CAD build for the part. Positions are in the model's coordinates, mm. Round coordinates to 2 decimals unless told otherwise and drop trailing zeros. Order: outer loops, then holes, each group sorted by start corner. A loop starts at its lowest first (then second) coordinate and runs counter-clockwise, first axis right, second up. Notation, with made-up numbers: (35.25, 7) -> (42.25, 7) arc R33 cw to (42.25, 44) -> close; hole circle Ø4 at (-31.75, -12). An arc over 180 degrees is marked (long way). Return JSON: item names as keys, results as strings. Group by question number.
Q1. Mould opens along Y. For faces 1 (the cylindrical face through (-4.119, 213.452, 1.479)), 2 (the flat face through (-9, 4, 0)) say: +Y half, -Y half, draft (parallel to the pull), parting line (faces both ways), or undercut.
Q2. Cut at B-B (x = 0). Write the cut outline in (y, z).
Q3. Cut at A-A (y = 232). Write the cut outline in (x, z), then the cut area to 3 significant figures.
Q4. Probe line 1 along Y through (x, z) = (-101, 2.2); line 2 along X through (y, z) = (-180, 0.8); line 3 along Y through (x, z) = (615, 2.15). List the from-to ranges inside material, lowest first.
Q5. Flat gauge pins, fed straight in: pin 1 (8 mm diameter, centred on x = -303, y = -290, fed in from -Z); pin 2 (4 mm diameter, centred on x = 101, y = -290, fed in from -Z). Where does each tip first touch, or does it go through?
from build123d import *

# Parameters (mm, degrees)
SKETCH1_W           = 1250
SKETCH1_H           = 600
SKETCH1_R           = 2.55
SKETCH1_R_2         = 19
BOSS_EXTRUDE1_DEPTH = 3


with BuildPart() as part:
    # Sketch1 → Boss-Extrude1 (new body)
    with BuildSketch(Plane.XY):
        Rectangle(SKETCH1_W, SKETCH1_H)
        with Locations((303, 290)):
            Circle(SKETCH1_R, mode=Mode.SUBTRACT)
        with Locations((101, 290)):
            Circle(SKETCH1_R, mode=Mode.SUBTRACT)
        with Locations((-101, 290)):
            Circle(SKETCH1_R, mode=Mode.SUBTRACT)
        with Locations((-303, 290)):
            Circle(SKETCH1_R, mode=Mode.SUBTRACT)
        with Locations((505, 290)):
            Circle(SKETCH1_R, mode=Mode.SUBTRACT)
        with Locations((505, -290)):
            Circle(SKETCH1_R, mode=Mode.SUBTRACT)
        with Locations((-505, 290)):
            Circle(SKETCH1_R, mode=Mode.SUBTRACT)
        with Locations((303, -290)):
            Circle(SKETCH1_R, mode=Mode.SUBTRACT)
        with Locations((101, -290)):
            Circle(SKETCH1_R, mode=Mode.SUBTRACT)
        with Locations((-101, -290)):
            Circle(SKETCH1_R, mode=Mode.SUBTRACT)
        with Locations((615, 180)):
            Circle(SKETCH1_R, mode=Mode.SUBTRACT)
        with Locations((-615, 180)):
            Circle(SKETCH1_R, mode=Mode.SUBTRACT)
        with Locations((-615, 0)):
            Circle(SKETCH1_R, mode=Mode.SUBTRACT)
        with Locations((-615, -180)):
            Circle(SKETCH1_R, mode=Mode.SUBTRACT)
        with Locations((-303, -290)):
            Circle(SKETCH1_R, mode=Mode.SUBTRACT)
        with Locations((615, 0)):
            Circle(SKETCH1_R, mode=Mode.SUBTRACT)
        with Locations((615, -180)):
            Circle(SKETCH1_R, mode=Mode.SUBTRACT)
        with Locations((-505, -290)):
            Circle(SKETCH1_R, mode=Mode.SUBTRACT)
        with Locations((0, 232)):
            Circle(SKETCH1_R_2, mode=Mode.SUBTRACT)
    extrude(amount=BOSS_EXTRUDE1_DEPTH)


solid = part.part
Solution:
{
 "1": {"face 1": "undercut", "face 2": "draft"},
 "2": {"outline": "(-300, 0) -> (213, 0) -> (213, 3) -> (-300, 3) -> close; (251, 0) -> (300, 0) -> (300, 3) -> (251, 3) -> close"},
 "3": {"outline": "(-625, 0) -> (-19, 0) -> (-19, 3) -> (-625, 3) -> close; (19, 0) -> (625, 0) -> (625, 3) -> (19, 3) -> close", "area": "3,640 mm²"},
 "4": {"line 1": "y = -300 to -292.55, -287.45 to 287.45, 292.55 to 300", "line 2": "x = -625 to -617.55, -612.45 to 612.45, 617.55 to 625", "line 3": "y = -300 to -182.55, -177.45 to -2.55, 2.55 to 177.45, 182.55 to 300"},
 "5": {"pin 1": "stops at z = 0", "pin 2": "passes through"}
}
